Work out the finished part from the listing and answer in its coordinate system (mm). Face numbers are marked on the shaded views. A direction names the side the tool comes from. Round coordinates to 2 decimals unless told otherwise and drop trailing zeros. Write each loop counter-clockwise with the first axis right and the second up, starting at its lowest first coordinate (ties: lowest second). Pieces come first, ordered by that corner, then holes.
1. Flat-ended cylindrical pins translate along their axes: pin 1 Ø1.5 at (y, z) = (-10.5, 2.5) entering from +X; pin 2 Ø2 at (y, z) = (-3, 4) entering from +X; pin 3 Ø2.5 at (x, z) = (-11, 2.5) entering from -Y; pin 4 Ø3 at (x, y) = (-13.21, 0) entering from -Z. Find the tip coordinate at first contact, or state that the pin passes through.
2. A tool of negligible diameter and unlimited length cuts with its end or side. For the marked faces 1, 2, 3, 4 and 5, from which of +Z, -Z, +X, -X, +Y, -Y can it reach the whole face along a straight path? Write none if from no direction.
3. Straight lines are drawn through the part: probe 1 along X at (y, z) = (-12.5, 0.5); probe 2 along X at (y, z) = (-16, 1.75); probe 3 along X at (y, z) = (1.5, -3.5). For each, find the intervals that lie inside material, in ascending order.
4. Find section A-A (y = 0). Write down the section's boundary in (x, z).
5. Find section B-B (z = -3.5). Write down the section's boundary in (x, y).
6. Determine the mould class of the marked faces 6, 7, 8 and 9 for opening direction X: pulls with the +X half, pulls with the -X half, needs draft (parallel to the pull), parting line crosses it, or undercut.
7. Find section C-C (x = 16). Write down the section's boundary in (y, z), and give its area (3 significant figures).
```python
from build123d import *

# Parameters (mm, degrees)
ESTRUSIONE_ESTRUSIONE3_DEPTH = 5
SCHIZZO3_R                   = 2.5
ESTRUSIONE_ESTRUSIONE4_DEPTH = 5
SCHIZZO7_W                   = 5
SCHIZZO7_H                   = 6
ESTRUSIONE_ESTRUSIONE5_DEPTH = 20
SCHIZZO6_R                   = 1.65
TAGLIO_ESTRUSIONE1_DEPTH     = 20
RACCORDO1_R                  = 2.5
SCHIZZO8_R                   = 1.25
TAGLIO_ESTRUSIONE2_DEPTH     = 38.469880381
RACCORDO2_R                  = 2
RACCORDO3_R                  = 10


with BuildPart() as part:
    # Schizzo1 → Estrusione-Estrusione3 (new body)
    with BuildSketch(Plane.XY):
        with BuildLine():
            Line((-13.207991803, 5), (16.792008197, 5))
            ThreePointArc((16.792008197, 5), (21.792008197, 0), (16.792008197, -5))
            Line((16.792008197, -5), (6.792008197, -5))
            Line((6.792008197, -5), (6.792008197, -18.794102079))
            Line((6.792008197, -18.794102079), (6.792008197, -28.794102079))
            Line((6.792008197, -28.794102079), (-3.207991803, -18.794102079))
            Line((-3.207991803, -18.794102079), (-3.207991803, -5))
            Line((-3.207991803, -5), (-13.207991803, -5))
            ThreePointArc((-13.207991803, -5), (-18.207991803, 0), (-13.207991803, 5))
        make_face()
    extrude(amount=ESTRUSIONE_ESTRUSIONE3_DEPTH)

    # Schizzo3 → Estrusione-Estrusione4 (add)
    with BuildSketch(Plane(origin=(0, 0, 0), x_dir=(-1, 0, 0), z_dir=(0, 0, -1))):
        with Locations(Location((-16.792008197, 0, 0), (0, 0, 180))):
            Circle(SCHIZZO3_R)
        with Locations(Location((13.207991803, 0, 0), (0, 0, 180))):
            Circle(SCHIZZO3_R)
    extrude(amount=ESTRUSIONE_ESTRUSIONE4_DEPTH)

    # Schizzo7 → Estrusione-Estrusione5 (add)
    with BuildSketch(Plane(origin=(17.793055138, -17.793055138, 0), x_dir=(0, 0, -1), z_dir=(-0.7071067811865562, 0.7071067811865389, 0))):
        with Locations((-2.5, 12.557829784)):
            Rectangle(SCHIZZO7_W, SCHIZZO7_H)
    extrude(amount=ESTRUSIONE_ESTRUSIONE5_DEPTH)

    # Schizzo6 → Taglio-Estrusione1 (cut)
    with BuildSketch(Plane(origin=(17.793055138, -17.793055138, 0), x_dir=(0, 0, -1), z_dir=(-0.7071067811865562, 0.7071067811865389, 0))):
        with Locations(Location((-2.5, 12.557829784, 0), (0, 0, 270))):
            Circle(SCHIZZO6_R)
    extrude(amount=TAGLIO_ESTRUSIONE1_DEPTH, mode=Mode.SUBTRACT)

    # Raccordo1
    raccordo1_edges = [part.edges().sort_by_distance(p)[0] for p in [
        (-0.279059615, -21.723034267, 0),
        (-0.279059615, -21.723034267, 5),
    ]]
    fillet(raccordo1_edges, radius=RACCORDO1_R - 0.0001)  # a hair under: the kernel refuses the full size

    # Schizzo8 → Taglio-Estrusione2 (cut, through all)
    with BuildSketch(Plane(origin=(0, 0, -5), x_dir=(-1, 0, 0), z_dir=(0, 0, -1))):
        with Locations((-16.792008197, 0)):
            Circle(SCHIZZO8_R)
        with Locations((13.207991803, 0)):
            Circle(SCHIZZO8_R)
    extrude(amount=-TAGLIO_ESTRUSIONE2_DEPTH, mode=Mode.SUBTRACT)

    # Raccordo2
    raccordo2_edges = [part.edges().sort_by_distance(p)[0] for p in [
        (6.792008197, -5, 2.5),
        (-3.207991803, -5, 2.5),
    ]]
    fillet(raccordo2_edges, radius=RACCORDO2_R)

    # Raccordo3
    raccordo3_edges = [part.edges().sort_by_distance(p)[0] for p in [
        (6.792008197, -20.308820704, 2.5),
    ]]
    fillet(raccordo3_edges, radius=RACCORDO3_R)


solid = part.part
```
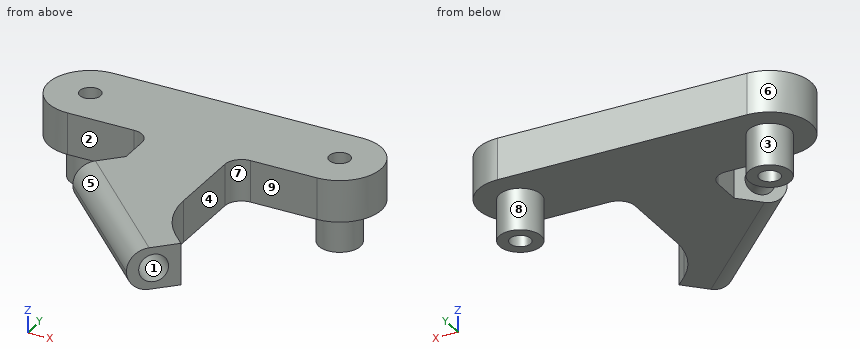
Worked answers:
1. pin 1: stops at x = 6.79
1. pin 2: stops at x = 21.37
1. pin 3: stops at y = -5
1. pin 4: stops at z = -5
2. face 1: none
2. face 2: +Z, -Z, -X
2. face 3: -Z
2. face 4: +Z, -Z, +X
2. face 5: +Z, -X, -Y
3. probe 1: x = -5.2 to 6.79
3. probe 2: x = -5.84 to -3.84, 0.32 to 6.79
3. probe 3: x = -15.21 to -11.21, 14.79 to 18.79
4. outline: (-18.21, 0) - (-15.71, 0) - (-15.71, -5) - (-14.46, -5) - (-14.46, 5) - (-18.21, 5) - close; (-11.96, -5) - (-10.71, -5) - (-10.71, 0) - (14.29, 0) - (14.29, -5) - (15.54, -5) - (15.54, 5) - (-11.96, 5) - close; (18.04, -5) - (19.29, -5) - (19.29, 0) - (21.79, 0) - (21.79, 5) - (18.04, 5) - close
5. outline: circle Ø5 at (-13.21, 0); circle Ø5 at (16.79, 0); hole circle Ø2.5 at (-13.21, 0); hole circle Ø2.5 at (16.79, 0)
6. face 6: pulls with the -X half
6. face 7: pulls with the +X half
6. face 8: undercut
6. face 9: needs draft
7. outline: (-5, 0) - (-2.37, 0) - (-2.37, -5) - (-0.97, -5) - (-0.97, 5) - (-5, 5) - close; (0.97, -5) - (2.37, -5) - (2.37, 0) - (5, 0) - (5, 5) - (0.97, 5) - close
7. area: 54.4 mm2
